Autodesk Inventor part; units mm, degrees
ref_plane "YZ Plane" through (0, 0, 0) normal (1, 0, 0) x (0, 1, 0)
ref_plane "XZ Plane" through (0, 0, 0) normal (0, 1, 0) x (-1, 0, 0)
ref_plane "XY Plane" through (0, 0, 0) normal (0, 0, 1) x (1, 0, 0)
sketch "Sketch1" plane through (0, 0, 0) normal (0, 1, 0) x (-1, 0, 0)
  line L0 (0, 5.08) -> (0, 10.668)
  line L1 (0, 0) -> (0, 10.668) construction
  line L2 (0, 10.668) -> (0, 18.542)
  line L3 (0, 18.542) -> (0, 24.13)
  line L4 (0, 24.13) -> (0, 32.004)
  line L5 (0, 32.004) -> (0, 37.592)
  line L6 (0, 37.592) -> (0, 45.466)
  line L7 (0, 45.466) -> (0, 51.054)
  line L8 (0, 51.054) -> (0, 58.928)
  line L9 (0, 58.928) -> (0, 66.802)
  line L10 (0, 0) -> (8.7387, 6.1189) construction
  line L11 (0, 0) -> (0, 18.542) construction
  line L12 (0, 0) -> (0, 24.13) construction
  line L13 (0, 0) -> (0, 32.004) construction
  line L14 (0, 0) -> (0, 37.592) construction
  line L15 (0, 0) -> (0, 45.466) construction
  line L16 (0, 0) -> (0, 51.054) construction
  line L17 (0, 0) -> (0, 58.928) construction
  line L18 (0, 0) -> (0, 66.802) construction
  line L19 (0, 0) -> (69.85, 0) construction
  line L20 (0, 0) -> (69.85, 0) construction
  line L21 (0, 66.802) -> (0, 69.85)
  line L22 (0, 0) -> (0, 5.08)
  line L23 (0, 69.85) -> (6.35, 69.85)
  line L24 (6.35, 69.85) -> (6.35, 0)
  line L25 (0, 5.08) -> (6.35, 5.08)
  line L26 (0, 10.668) -> (6.35, 10.668)
  line L27 (0, 18.542) -> (6.35, 18.542)
  line L28 (0, 24.13) -> (6.35, 24.13)
  line L29 (0, 32.004) -> (6.35, 32.004)
  line L30 (0, 37.592) -> (6.35, 37.592)
  line L31 (0, 45.466) -> (6.35, 45.466)
  line L32 (0, 51.054) -> (6.35, 51.054)
  line L33 (0, 58.928) -> (6.35, 58.928)
  dimension "d2" = 5.588
  dimension "d4" = 7.874
  dimension "d5" = 5.588
  dimension "d6" = 7.874
  dimension "d7" = 5.588
  dimension "d8" = 7.874
  dimension "d9" = 5.588
  dimension "d10" = 7.874
  dimension "d11" = 7.874
  dimension "d24" = 5.08
  dimension "d25" = 6.35
  dimension "d26" = 3.048
revolve "Revolution1" add sketch "Sketch1" angle 360 about axis through (0, 0, 0) along (-1, 0, 0) contours L0 L26 L24 L25 | L3 L28 L24 L27 | L5 L30 L24 L29 | L7 L32 L24 L31 | L9 L21 L23 L24 L33
sketch "Sketch2" plane through (-6.35, 0, 0) normal (-1, 0, 0) x (0, 0, 1)
  line L0 (69.6277, 3.175) -> (-69.6277, 3.175)
  line L1 (-69.6277, 3.175) -> (-69.6277, -3.175)
  line L2 (-69.6277, -3.175) -> (69.6277, -3.175)
  line L3 (69.6277, -3.175) -> (69.6277, 3.175)
  circle A0 centre (0, 0) radius 5.08
  line L4 (69.6277, 3.175) -> (-69.6277, -3.175) construction
  line L5 (-69.6277, 3.175) -> (69.6277, -3.175) construction
  line L6 (32.0642, 61.8868) -> (-37.5635, -58.7118)
  line L7 (-32.0642, -61.8868) -> (37.5635, 58.7118)
  line L8 (-37.5635, -58.7118) -> (-32.0642, -61.8868)
  line L9 (37.5635, 58.7118) -> (32.0642, 61.8868)
  line L10 (37.5635, -58.7118) -> (-32.0642, 61.8868)
  line L11 (-37.5635, 58.7118) -> (32.0642, -61.8868)
  line L12 (-32.0642, 61.8868) -> (-37.5635, 58.7118)
  line L13 (32.0642, -61.8868) -> (37.5635, -58.7118)
  point P0 (-5.4993, 3.175)
  point P1 (-5.4993, -3.175)
  point P2 (0, -6.35)
  point P3 (5.4993, -3.175)
  point P4 (5.4993, 3.175)
  point P5 (0, 6.35)
  dimension "d28" = 6.35
  dimension "d31" = 360
extrude "Extrusion1" add sketch "Sketch2" against normal blind 6.35
sketch "Sketch3" plane through (0, 0, 0) normal (1, 0, 0) x (0, 0, -1)
  circle A0 centre (0, 0) radius 5.08
  dimension "d35" = 10.16
extrude "Extrusion2" cut sketch "Sketch3" against normal blind 25.4
equation "\"d2\" = PR"
equation "\"d4\" = HR"
equation "\"d5\" = PR"
equation "\"d6\" = HR"
equation "\"d7\" = PR"
equation "\"d8\" = HR"
equation "\"d9\" = PR"
equation "\"d10\" = HR"
equation "\"d11\" = HR"
equation "\"HR\" = 7.874"
equation "\"PR\" = 5.588"
equation "\"HA\" = 55deg"
properties part number "flat drain cover"
CAD build for the part. Positions are in the model's coordinates, mm. Give positions to 0.01 mm unless a question says otherwise; leave off trailing zeros. Write each loop counter-clockwise with the first axis right and the second up, starting at its lowest first coordinate (ties: lowest second). Pieces come first, ordered by that corner, then holes. Notation, with made-up numbers: (14.25, 13.5) -> (40.25, 13.5) arc R4 cw to (40.25, 17.5) -> close; hole circle Ø1 at (8.5, 85). An arc over 180 degrees is marked (long way). Write each question's results on one line, items separated by ' | '.
1. Cut at A-A, the plane y = 0. Write the cut outline in (x, z), then the cut area to 3 significant figures.
Geometry check:
outline: (-6.35, -69.85) -> (0, -69.85) -> (0, -5.08) -> (-6.35, -5.08) -> close; (-6.35, 5.08) -> (0, 5.08) -> (0, 69.85) -> (-6.35, 69.85) -> close | area: 823 mm²
2. Cut at C-C, the plane z = 0. Give the number of separate pieces and of enclosed holes in the cut face, then the cut area to 3 significant figures.
Geometry check:
separate pieces: 10 | enclosed holes: 0 | area: 423 mm²
3. Cut at D-D, the plane z = -55.5. Write the cut outline in (x, y) (3 decimals).
Geometry check:
outline: (-6.35, -42.412) -> (0, -42.412) -> (0, -19.806) -> (-6.35, -19.806) -> close; (-6.35, -3.175) -> (0, -3.175) -> (0, 3.175) -> (-6.35, 3.175) -> close; (-6.35, 19.806) -> (0, 19.806) -> (0, 42.412) -> (-6.35, 42.412) -> close
4. Two-plate mould, pull along Y, no slides. Class faces 1 (the flat face through (0, 1, 15)), 2 (the cylindrical face through (-3.22, 25.81, -44.05)): pulls with the +Y half, pulls with the -Y half, needs draft (parallel to the pull), parting line crosses it, or undercut.
Geometry check:
face 1: needs draft | face 2: undercut
5. Wall check: probe 1 along Z at (x, y) = (-0.75, 42); probe 2 along Y at (x, z) = (-3, 54) (3 decimals); probe 3 along Y at (x, z) = (-1.75, -59). Give the ranges that are in metal, low to high. Write a range as [from, to].
Geometry check:
probe 1: [-55.81, -41.33], [-29.03, -17.41], [17.41, 29.03], [41.33, 55.81] | probe 2: [-44.306, -23.59], [-3.175, 3.175], [23.59, 44.306] | probe 3: [-37.39, 37.39]
6. Cut at B-B, the plane z = 34. Write the cut outline in (x, y).
Geometry check:
outline: (-6.35, -61.02) -> (0, -61.02) -> (0, -48.13) -> (-6.35, -48.13) -> close; (-6.35, -38.09) -> (0, -38.09) -> (0, -30.19) -> (-6.35, -30.19) -> close; (-6.35, -16.04) -> (0, -16.04) -> (0, 16.04) -> (-6.35, 16.04) -> close; (-6.35, 30.19) -> (0, 30.19) -> (0, 38.09) -> (-6.35, 38.09) -> close; (-6.35, 48.13) -> (0, 48.13) -> (0, 61.02) -> (-6.35, 61.02) -> close
7. Drop flat-ended pins along their axis: P1, Ø1.9, axis at x = -2, z = 28, coming from the -Y side; P2, Ø3, axis at y = -41.5, z = 20, coming from the +X side; P3, Ø1.5, axis at x = -2.5, y = -8, coming from the -Z side; P4, Ø1, axis at y = 19, z = -34, coming from the -X side. Give the stop position or say it passes through.
Geometry check:
P1: y = -64.4 | P2: x = 0 | P3: z = -69.47 | P4: through
